CAD build for the part. Positions are in the model's coordinates, mm. A direction names the side the tool comes from. Coordinates: 2 decimals unless noted, no trailing zeros. Order: outer loops, then holes, each group sorted by start corner. A loop starts at its lowest first (then second) coordinate and runs counter-clockwise, first axis right, second up. Notation, with made-up numbers: (-9.75, -18.75) - (41.25, -18.75) arc R21 cw to (41.25, -13.75) - close; hole circle Ø7 at (26.5, 40.5). An arc over 180 degrees is marked (long way). Return JSON: item names as keys, results as strings.
Autodesk Inventor part; units mm, degrees
ref_plane "Start plane" through (0, 0, 30) normal (0, 0, 1) x (1, 0, 0)
ref_plane "End plane" through (0, 0, 350) normal (0, 0, 1) x (1, 0, 0)
ref_plane "Work Plane4" through (599.2, 515, 350) normal (0, 0, 1) x (1, 0, 0)
ref_plane "Start plane" through (0, 0, 30) normal (0, 0, 1) x (1, 0, 0)
ref_plane "End plane" through (0, 0, 350) normal (0, 0, 1) x (1, 0, 0)
sketch "Sketch" plane through (0, 0, 0) normal (0, 0, 1) x (1, 0, 0)
  line L0 (-15, -11.25) -> (-15, 11.25)
  line L1 (-11.25, 15) -> (11.25, 15)
  line L2 (15, 11.25) -> (15, -11.25)
  line L3 (11.25, -15) -> (-11.25, -15)
  arc A0 (-15, -11.25) -> (-11.25, -15) centre (-11.25, -11.25) ccw
  arc A1 (-11.25, 15) -> (-15, 11.25) centre (-11.25, 11.25) ccw
  arc A2 (15, 11.25) -> (11.25, 15) centre (11.25, 11.25) ccw
  arc A3 (11.25, -15) -> (15, -11.25) centre (11.25, -11.25) ccw
  arc A4 (-11.25, 12.5) -> (-12.5, 11.25) centre (-11.25, 11.25) ccw
  line L4 (-11.25, 12.5) -> (11.25, 12.5)
  arc A5 (12.5, 11.25) -> (11.25, 12.5) centre (11.25, 11.25) ccw
  line L5 (12.5, 11.25) -> (12.5, -11.25)
  arc A6 (11.25, -12.5) -> (12.5, -11.25) centre (11.25, -11.25) ccw
  line L6 (11.25, -12.5) -> (-11.25, -12.5)
  arc A7 (-12.5, -11.25) -> (-11.25, -12.5) centre (-11.25, -11.25) ccw
  line L7 (-12.5, -11.25) -> (-12.5, 11.25)
  line L8 (0, 22.0873) -> (0, -22.0873) construction
  line L9 (-22.0873, 0) -> (22.0873, 0) construction
  dimension "d7" = 3.75
  dimension "d10" = 30
  dimension "d11" = 30
  dimension "d12" = 2.5
  dimension "d15" = 15
  dimension "d16" = 15
extrude "Body" add sketch "Sketch" along normal up to surface (320 mm away) from surface at 30
sketch "Sketch3" plane through (0, 0, 0) normal (0, 0, 1) x (1, 0, 0)
  line L0 (0, 0) -> (10, 0)
ref_plane "Work Plane3" through (0, 0, 0) normal (0, -1, 0) x (1, 0, 0)
sketch "Sketch4" plane through (0, 0, 0) normal (0, -1, 0) x (1, 0, 0)
  line L0 (-2, 30) -> (12, 30)
  line L1 (-2, 350) -> (12, 350)
  dimension "d18" = 320
ref_plane "Work Plane4" through (599.2, 515, 350) normal (0, 0, 1) x (1, 0, 0)
split "Split1" plane through (599.2, 515, 350) removes the side toward (0, 0, 1)
ref_plane "Work Plane5" through (-15, -11.25, 30) normal (0, 0, -1) x (-1, 0, 0)
split "Split2" plane through (-15, -11.25, 30) removes the side toward (0, 0, -1)
equation "\"d7\" = G_IR"
equation "\"d10\" = G_H"
equation "\"d11\" = G_W"
equation "\"d12\" = G_T"
equation "\"d15\" = 0.5 * d10"
equation "\"d16\" = 0.5 * d11"
equation "\"d3\" = G_L"
equation "\"G_W\" = 30"
equation "\"G_H\" = 30"
equation "\"G_T\" = 2.5"
equation "\"G_IR\" = 3.75"
equation "\"G_L\" = d18"
properties part number "DIN EN 10305-5 - 30 x 30 x 2,5  - 320" material "Steel, Mild"
Item 1: Which spindle directions (+Z, -Z, +X, -X, +Y, -Y) get a long thin tool onto all of the face, cutting with end or side? Do faces 1 (the flat face through (0, -15, 188)), 2 (the flat face through (12.5, 0, 188)). Say none if no direction does.
Findings below:
{"face 1": "+Z, -Z, +X, -X, -Y", "face 2": "+Z, -Z"}
Item 2: Wall check: L1, parallel to X at y = -8.25, z = 226; L2, parallel to Y at x = 13.75, z = 272. Give the ranges that are in metal, low to high. Write a range as [from, to].
Findings below:
{"L1": "x = [-15, -12.5], [12.5, 15]", "L2": "y = [-14.05, 14.05]"}
Item 3: Drop flat-ended pins along their axis: P1, Ø8, axis at x = -12, z = 66, coming from the -Y side; P2, Ø1.5, axis at x = 7, y = 10, coming from the -Z side. Give the stop position or say it passes through.
Findings below:
{"P1": "stops at y = -15", "P2": "passes through"}
Item 4: Band-saw the part on B-B, the plane z = 272. List the corners of the cut face in (x, y), then the cut area to 3 significant figures.
Findings below:
{"outline": "(-15, -11.25) arc R3.75 ccw to (-11.25, -15) - (11.25, -15) arc R3.75 ccw to (15, -11.25) - (15, 11.25) arc R3.75 ccw to (11.25, 15) - (-11.25, 15) arc R3.75 ccw to (-15, 11.25) - close; hole (-12.5, -11.25) arc R1.25 ccw to (-11.25, -12.5) - (11.25, -12.5) arc R1.25 ccw to (12.5, -11.25) - (12.5, 11.25) arc R1.25 ccw to (11.25, 12.5) - (-11.25, 12.5) arc R1.25 ccw to (-12.5, 11.25) - close", "area": "264 mm²"}
Item 5: Band-saw the part on A-A, the plane y = 8.5. List the corners of the cut face in (x, z), then the cut area to 3 significant figures.
Findings below:
{"outline": "(-15, 30) - (-12.5, 30) - (-12.5, 350) - (-15, 350) - close; (12.5, 30) - (15, 30) - (15, 350) - (12.5, 350) - close", "area": "1,600 mm²"}
